Geometry check sheet. Reference: the model listing, model coordinates, mm. Face numbers are marked on the shaded views. A direction names the side the tool comes from. Coordinates: 2 decimals unless noted, no trailing zeros. Write each loop counter-clockwise with the first axis right and the second up, starting at its lowest first coordinate (ties: lowest second). Pieces come first, ordered by that corner, then holes. Notation, with made-up numbers: (-15.75, 36) -> (34.25, 36) arc R29 cw to (34.25, 59) -> close; hole circle Ø11 at (-30, -2.75). An arc over 180 degrees is marked (long way). Answer in a Markdown table with one row per item. Add a question column.
Q1. Thickness scan on line 1 (Y direction, x = 5, z = 19); line 2 (Y direction, x = 6, z = 11.25). Record the ranges inside material, lowest first.
Q2. Gauge pin test, flat ends, axial feed: P1, Ø8, axis at y = 4.5, z = 2, coming from the -X side; P2, Ø2, axis at x = -0.5, z = 5.5, coming from the -Y side; P3, Ø5, axis at x = -3.5, z = 9, coming from the -Y side. Record the tip position at first contact, or that the pin passes through.
Q3. Section check A-A, the plane z = 4.5. Record the boundary of the cut face in (x, y), and give its area (3 significant figures).
Q4. Release check for a two-part mould opening along X. For the marked faces 4, 5 and 6 record: pulls with the +X half, pulls with the -X half, needs draft (parallel to the pull), parting line crosses it, or undercut.
Q5. Section check B-B, the plane x = 3.5. Record the boundary of the cut face in (y, z).
Q6. Tool access check on the marked faces 1, 2 and 3. Record the directions out of +Z, -Z, +X, -X, +Y, -Y that give a thin tool (end or side, any length) a straight path to the whole face; none if there is none.
Autodesk Inventor part; units mm, degrees
ref_plane "YZ Plane" through (0, 0, 0) normal (1, 0, 0) x (0, 1, 0)
ref_plane "XZ Plane" through (0, 0, 0) normal (0, 1, 0) x (-1, 0, 0)
ref_plane "XY Plane" through (0, 0, 0) normal (0, 0, 1) x (1, 0, 0)
sketch "Sketch1" plane through (0, 0, 0) normal (0, 0, 1) x (1, 0, 0)
  circle A0 centre (0, 0) radius 2.5
  dimension "d0" = 5
extrude "Extrusion1" add sketch "Sketch1" along normal blind 10
sketch "Sketch2" plane through (0, 0, 10) normal (0, 0, 1) x (1, 0, 0)
  circle A0 centre (0, 0) radius 6.99
  circle A1 centre (0, 0) radius 4.85
  line L0 (-6.99, 0) -> (6.99, 0)
  arc A2 (6.9831, 0.31) -> (4.7977, 0.71) centre (5.4872, -1.6931) ccw
  arc A3 (4.7977, -0.71) -> (6.9831, -0.31) centre (5.4872, 1.6931) ccw
  point P0 (4.8336, 0.3987)
  point P1 (4.7977, -0.71)
  point P2 (6.9831, -0.31)
  dimension "d3" = 13.98
  dimension "d17" = 9.7
  dimension "d18" = 0.62
  dimension "d19" = 1.42
  dimension "d20" = 2.5
extrude "Extrusion2" add sketch "Sketch2" along normal blind 10 contours L0 A1 | A1 L0
extrude "Extrusion3" add sketch "Sketch2" along normal up to surface (10 mm away) contours L0 A1 A2 A0 | A0 A3 A1 L0 | L0 A1 | A1 L0 picked at (6.1088, 0.1995) picked at (6.1089, -0.1995)
pattern_circular "Circular Pattern1" count 12 over 360 about axis through (0, 0, -10) along (0, 0, 1) of "Extrusion3"
sketch "Sketch3" plane through (0, 0, 20) normal (0, 0, 1) x (1, 0, 0)
  line L0 (-2.04, -2.04) -> (2.04, -2.04)
  line L1 (2.04, -2.04) -> (2.04, 2.04)
  line L2 (2.04, 2.04) -> (-2.04, 2.04)
  line L3 (-2.04, 2.04) -> (-2.04, -2.04)
  line L4 (-2.04, -2.04) -> (2.04, 2.04) construction
  line L5 (2.04, -2.04) -> (-2.04, 2.04) construction
  point P0 (0, 0)
  dimension "d22" = 4.08
extrude "Extrusion4" cut sketch "Sketch3" against normal through all
properties part number "Pinion Gear"
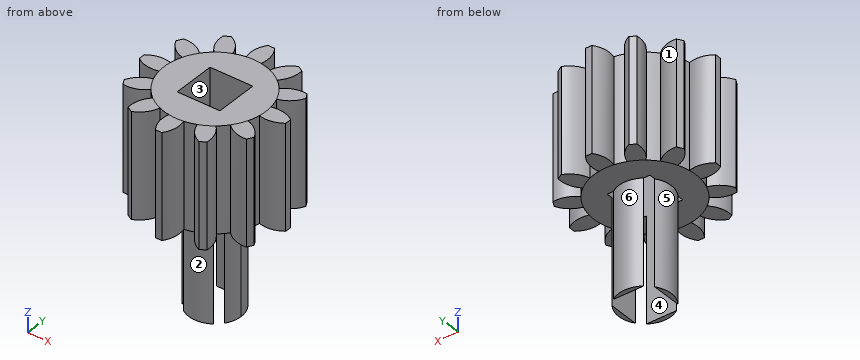
Calculated:
| question | item | result |
|---|---|---|
| 1 | line 1 | y = -3.7 to -1.96, -0.76 to 0.76, 1.96 to 3.7 |
| 1 | line 2 | y = -3.59 to -2.84, -0.75 to 0.75, 2.84 to 3.59 |
| 2 | P1 | stops at x = -2.45 |
| 2 | P2 | stops at y = -2.5 |
| 2 | P3 | stops at y = -6.2 |
| 3 | outline | (-2.04, -1.45) -> (-2.04, 1.45) arc R2.5 ccw to start; (-1.45, -2.04) arc R2.5 ccw to (1.45, -2.04) -> close; (-1.45, 2.04) -> (1.45, 2.04) arc R2.5 ccw to start; (2.04, -1.45) arc R2.5 ccw to (2.04, 1.45) -> close |
| 3 | area | 3.62 mm² |
| 4 | face 4 | undercut |
| 4 | face 5 | pulls with the -X half |
| 4 | face 6 | parting line crosses it |
| 5 | outline | (-6.05, 10) -> (-4.45, 10) -> (-4.45, 20) -> (-6.05, 20) -> close; (-3.36, 10) -> (3.36, 10) -> (3.36, 20) -> (-3.36, 20) -> close; (4.45, 10) -> (6.05, 10) -> (6.05, 20) -> (4.45, 20) -> close |
| 6 | face 1 | +Z, -Z, +Y |
| 6 | face 2 | -Z, -Y |
| 6 | face 3 | +Z, -Z |
